```python
from build123d import *

# Parameters (mm, degrees)
SKETCH1_W                       = 46
SKETCH1_H                       = 95.52
BOSS_EXTRUDE1_DEPTH             = 3.175
SKETCH2_W                       = 20
SKETCH2_H                       = 30.52
CUT_EXTRUDE1_DEPTH              = 54.104597023
F_6_0MM_CLEARANCE_DOWEL_HOLE1_D = 6
F_6_0MM_DOWEL_HOLE1_D           = 6
CUT_EXTRUDE2_DEPTH              = 54.104597023
SKETCH10_W                      = 21.52
SKETCH10_H                      = 8.52
CUT_EXTRUDE3_DEPTH              = 54.104597023
SKETCH11_W                      = 21.52
SKETCH11_H                      = 25
CUT_EXTRUDE4_DEPTH              = 54.104597023
SKETCH14_R                      = 3
CUT_EXTRUDE5_DEPTH              = 54.104597023


with BuildPart() as part:
    # Sketch1 → Boss-Extrude1 (new body)
    with BuildSketch(Plane(origin=(0, 0, 0), x_dir=(0, 0, -1), z_dir=(1, 0, 0))):
        Rectangle(SKETCH1_W, SKETCH1_H)
    extrude(amount=BOSS_EXTRUDE1_DEPTH)

    # Sketch2 → Cut-Extrude1 (cut, through all)
    with BuildSketch(Plane(origin=(3.175, 0, 0), x_dir=(0, 0, -1), z_dir=(1, 0, 0))):
        with Locations((13, 20.5)):
            Rectangle(SKETCH2_W, SKETCH2_H)
    extrude(amount=-CUT_EXTRUDE1_DEPTH, mode=Mode.SUBTRACT)

    # Ø6.0mm Clearance Dowel Hole1 (through all)
    with Locations(Plane(origin=(3.175, 0, 0), x_dir=(0, 0, -1), z_dir=(1, 0, 0))):
        with Locations((17, -2.76), (17, -39.76)):
            Hole(F_6_0MM_CLEARANCE_DOWEL_HOLE1_D / 2)

    # Ø6.0mm Dowel Hole1 (through all)
    with Locations(Plane(origin=(3.175, 0, 0), x_dir=(0, 0, -1), z_dir=(1, 0, 0))):
        with Locations((17, 41.76), (-17, 41.76), (-17, -39.76)):
            Hole(F_6_0MM_DOWEL_HOLE1_D / 2)

    # Sketch9 → Cut-Extrude2 (cut, through all)
    with BuildSketch(Plane(origin=(3.175, 0, 0), x_dir=(0, 0, -1), z_dir=(1, 0, 0))):
        Polygon((3, 35.76), (0.701902961, 33.461902961), (0.701902961, 5.24), (3, 5.24), align=None)
    extrude(amount=-CUT_EXTRUDE2_DEPTH, mode=Mode.SUBTRACT)

    # Sketch10 → Cut-Extrude3 (cut, through all)
    with BuildSketch(Plane(origin=(3.175, 0, 0), x_dir=(0, 0, -1), z_dir=(1, 0, 0))):
        with Locations((0, 0.98)):
            Rectangle(SKETCH10_W, SKETCH10_H)
    extrude(amount=-CUT_EXTRUDE3_DEPTH, mode=Mode.SUBTRACT)

    # Sketch11 → Cut-Extrude4 (cut, through all)
    with BuildSketch(Plane(origin=(3.175, 0, 0), x_dir=(0, 0, -1), z_dir=(1, 0, 0))):
        with Locations((0, -15.78)):
            Rectangle(SKETCH11_W, SKETCH11_H)
    extrude(amount=-CUT_EXTRUDE4_DEPTH, mode=Mode.SUBTRACT)

    # Sketch14 → Cut-Extrude5 (cut, through all)
    with BuildSketch(Plane(origin=(3.175, 0, 0), x_dir=(0, 0, -1), z_dir=(1, 0, 0))):
        with Locations((-16.76, 0.39)):
            Circle(SKETCH14_R)
        with BuildLine():
            Line((-13.76, -9.77), (-13.76, -19.77))
            ThreePointArc((-13.76, -19.77), (-16.76, -22.77), (-19.76, -19.77))
            Line((-19.76, -19.77), (-19.76, -9.77))
            ThreePointArc((-19.76, -9.77), (-16.76, -6.77), (-13.76, -9.77))
        make_face()
    extrude(amount=-CUT_EXTRUDE5_DEPTH, mode=Mode.SUBTRACT)


solid = part.part
```
Could you check a few things on this model? Use its own coordinates, in mm. A direction names the side the tool comes from. Coordinates: 2 decimals unless noted, no trailing zeros. Write each loop counter-clockwise with the first axis right and the second up, starting at its lowest first coordinate (ties: lowest second). Pieces come first, ordered by that corner, then holes. Notation, with made-up numbers: (-36, 6.25) -> (17, 6.25) arc R30 cw to (17, 41.25) -> close; hole circle Ø10 at (63.25, 5.5). An arc over 180 degrees is marked (long way). Return JSON: item names as keys, results as strings.
(1) Which directions (+Z, -Z, +X, -X, +Y, -Y) give clear straight access to the entire face, cutting with the end or side of a thin tool? Please do faces 4 (the flat face through (1.61, 34.63, -1.87)), 5 (the flat face through (0, 11, 0)), 6 (the cylindrical face through (1.61, -22.77, 16.69)).
Numbers:
{"face 4": "-Z, +X, -X", "face 5": "+Z, -Z, -X, +Y, -Y", "face 6": "+X, -X"}
(2) Imagine slicing it at C-C, the plane x = 1.45. Please give me the cut outline in (y, z), then the cut area to 3 significant figures.
Numbers:
{"outline": "(-47.76, -23) -> (5.24, -23) -> (5.24, -10.76) -> (-28.28, -10.76) -> (-28.28, 10.76) -> (5.24, 10.76) -> (5.24, -0.7) -> (33.46, -0.7) -> (35.76, -3) -> (35.76, -23) -> (47.76, -23) -> (47.76, 23) -> (-47.76, 23) -> close; hole circle Ø6 at (-39.76, -17); hole circle Ø6 at (-39.76, 17); hole (-19.77, 13.76) -> (-9.77, 13.76) arc R3 ccw to (-9.77, 19.76) -> (-19.77, 19.76) arc R3 ccw to start; hole circle Ø6 at (-2.76, -17); hole circle Ø6 at (0.39, 16.76); hole circle Ø6 at (41.76, -17); hole circle Ø6 at (41.76, 17)", "area": "2,740 mm2"}
(3) We'd pull the mould along Y, two halves only. Please class faces 1 (the flat face through (2, -47.76, 0)), 2 (the cylindrical face through (1.57, 38.83, 16.35)), 3 (the flat face through (2, -1, 23)): +Y half, -Y half, draft (parallel to the pull), parting line (faces both ways), or undercut.
Numbers:
{"face 1": "-Y half", "face 2": "undercut", "face 3": "draft"}
(4) Imagine slicing it at A-A, the plane z = -7. Please give me the cut outline in (x, y) (3 decimals).
Numbers:
{"outline": "(0, -47.76) -> (3.175, -47.76) -> (3.175, -28.28) -> (0, -28.28) -> close; (0, 35.76) -> (3.175, 35.76) -> (3.175, 47.76) -> (0, 47.76) -> close"}
(5) Imagine slicing it at D-D, the plane z = 2. Please give me the cut outline in (x, y) (3 decimals).
Numbers:
{"outline": "(0, -47.76) -> (3.175, -47.76) -> (3.175, -28.28) -> (0, -28.28) -> close; (0, 5.24) -> (3.175, 5.24) -> (3.175, 47.76) -> (0, 47.76) -> close"}
(6) Imagine slicing it at B-B, the plane y = -39.76. Please give me the cut outline in (x, z) (3 decimals).
Numbers:
{"outline": "(0, -23) -> (3.175, -23) -> (3.175, -20) -> (0, -20) -> close; (0, -14) -> (3.175, -14) -> (3.175, 14) -> (0, 14) -> close; (0, 20) -> (3.175, 20) -> (3.175, 23) -> (0, 23) -> close"}
(7) I'm going to push flat-ended pins straight in: pin 1 (8 mm diameter, centred on y = 0.39, z = 16.76, fed in from +X) (3 decimals); pin 2 (1 mm diameter, centred on x = 1.5, y = 17, fed in from -Z). Where does each tip first touch, or does it pass through?
Numbers:
{"pin 1": "stops at x = 3.175", "pin 2": "stops at z = -0.7"}
(8) I need wall thicknesses on L1, parallel to Z at x = 2.7, y = -14; L2, parallel to Y at x = 1.5, z = 16.76; L3, parallel to Y at x = 1, z = -17. Which ranges of each line are inside material? Lowest first, please.
Numbers:
{"L1": "z = -23 to -10.76, 10.76 to 13.76, 19.76 to 23", "L2": "y = -47.76 to -42.75, -36.77 to -22.77, -6.77 to -2.61, 3.39 to 38.77, 44.75 to 47.76", "L3": "y = -47.76 to -42.76, -36.76 to -5.76, 0.24 to 5.24, 35.76 to 38.76, 44.76 to 47.76"}
